Can you work these out from the model? Positions are in its coordinate system, mm. Round coordinates to 2 decimals unless told otherwise and drop trailing zeros. Return JSON: item names as keys, results as strings.
```python
from build123d import *

# Parameters (mm, degrees)
SKETCH_1_R      = 3.4
SKETCH_1_R_2    = 2
EXTRUDE_1_DEPTH = 1000


with BuildPart() as part:
    # 草图1 → 凸台-拉伸1 (new body)
    with BuildSketch(Plane.XY):
        with BuildLine():
            Line((5.39426949, 3.798904284), (9.399904408, 7.804539202))
            Line((9.399904408, 7.804539202), (12.09426949, 7.804539202))
            ThreePointArc((12.09426949, 7.804539202), (12.306401524, 7.716671237), (12.39426949, 7.504539202))
            Line((12.39426949, 7.504539202), (12.39426949, 3.954539202))
            ThreePointArc((12.39426949, 3.954539202), (12.482137455, 3.742407168), (12.69426949, 3.654539202))
            Line((12.69426949, 3.654539202), (13.59426949, 3.654539202))
            Line((13.59426949, 3.654539202), (13.59426949, 4.454539202))
            ThreePointArc((13.59426949, 4.454539202), (13.652848133, 4.595960558), (13.79426949, 4.654539202))
            Line((13.79426949, 4.654539202), (14.59426949, 4.654539202))
            Line((14.59426949, 4.654539202), (14.59426949, 12.054539202))
            ThreePointArc((14.59426949, 12.054539202), (13.862036443, 13.822306155), (12.09426949, 14.554539202))
            Line((12.09426949, 14.554539202), (4.69426949, 14.554539202))
            Line((4.69426949, 14.554539202), (4.69426949, 13.754539202))
            ThreePointArc((4.69426949, 13.754539202), (4.635690846, 13.613117846), (4.49426949, 13.554539202))
            Line((4.49426949, 13.554539202), (3.69426949, 13.554539202))
            Line((3.69426949, 13.554539202), (3.69426949, 12.654539202))
            ThreePointArc((3.69426949, 12.654539202), (3.782137455, 12.442407168), (3.99426949, 12.354539202))
            Line((3.99426949, 12.354539202), (7.54426949, 12.354539202))
            ThreePointArc((7.54426949, 12.354539202), (7.756401524, 12.266671237), (7.84426949, 12.054539202))
            Line((7.84426949, 12.054539202), (7.84426949, 9.360174121))
            Line((7.84426949, 9.360174121), (3.838634571, 5.354539202))
            Line((3.838634571, 5.354539202), (-4.650095592, 5.354539202))
            Line((-4.650095592, 5.354539202), (-8.65573051, 9.360174121))
            Line((-8.65573051, 9.360174121), (-8.65573051, 12.054539202))
            ThreePointArc((-8.65573051, 12.054539202), (-8.567862545, 12.266671237), (-8.35573051, 12.354539202))
            Line((-8.35573051, 12.354539202), (-4.80573051, 12.354539202))
            ThreePointArc((-4.80573051, 12.354539202), (-4.593598476, 12.442407168), (-4.50573051, 12.654539202))
            Line((-4.50573051, 12.654539202), (-4.50573051, 13.554539202))
            Line((-4.50573051, 13.554539202), (-5.30573051, 13.554539202))
            ThreePointArc((-5.30573051, 13.554539202), (-5.447151867, 13.613117846), (-5.50573051, 13.754539202))
            Line((-5.50573051, 13.754539202), (-5.50573051, 14.554539202))
            Line((-5.50573051, 14.554539202), (-12.90573051, 14.554539202))
            ThreePointArc((-12.90573051, 14.554539202), (-14.673497463, 13.822306155), (-15.40573051, 12.054539202))
            Line((-15.40573051, 12.054539202), (-15.40573051, 4.654539202))
            Line((-15.40573051, 4.654539202), (-14.60573051, 4.654539202))
            ThreePointArc((-14.60573051, 4.654539202), (-14.464309154, 4.595960558), (-14.40573051, 4.454539202))
            Line((-14.40573051, 4.454539202), (-14.40573051, 3.654539202))
            Line((-14.40573051, 3.654539202), (-13.50573051, 3.654539202))
            ThreePointArc((-13.50573051, 3.654539202), (-13.293598476, 3.742407168), (-13.20573051, 3.954539202))
            Line((-13.20573051, 3.954539202), (-13.20573051, 7.504539202))
            ThreePointArc((-13.20573051, 7.504539202), (-13.117862545, 7.716671237), (-12.90573051, 7.804539202))
            Line((-12.90573051, 7.804539202), (-10.211365429, 7.804539202))
            Line((-10.211365429, 7.804539202), (-6.20573051, 3.798904284))
            Line((-6.20573051, 3.798904284), (-6.20573051, -4.689825879))
            Line((-6.20573051, -4.689825879), (-10.211365429, -8.695460798))
            Line((-10.211365429, -8.695460798), (-12.90573051, -8.695460798))
            ThreePointArc((-12.90573051, -8.695460798), (-13.117862545, -8.607592832), (-13.20573051, -8.395460798))
            Line((-13.20573051, -8.395460798), (-13.20573051, -4.845460798))
            ThreePointArc((-13.20573051, -4.845460798), (-13.293598476, -4.633328763), (-13.50573051, -4.545460798))
            Line((-13.50573051, -4.545460798), (-14.40573051, -4.545460798))
            Line((-14.40573051, -4.545460798), (-14.40573051, -5.345460798))
            ThreePointArc((-14.40573051, -5.345460798), (-14.464309154, -5.486882154), (-14.60573051, -5.545460798))
            Line((-14.60573051, -5.545460798), (-15.40573051, -5.545460798))
            Line((-15.40573051, -5.545460798), (-15.40573051, -12.945460798))
            ThreePointArc((-15.40573051, -12.945460798), (-14.673497463, -14.713227751), (-12.90573051, -15.445460798))
            Line((-12.90573051, -15.445460798), (-5.50573051, -15.445460798))
            Line((-5.50573051, -15.445460798), (-5.50573051, -14.645460798))
            ThreePointArc((-5.50573051, -14.645460798), (-5.447151867, -14.504039442), (-5.30573051, -14.445460798))
            Line((-5.30573051, -14.445460798), (-4.50573051, -14.445460798))
            Line((-4.50573051, -14.445460798), (-4.50573051, -13.545460798))
            ThreePointArc((-4.50573051, -13.545460798), (-4.593598476, -13.333328763), (-4.80573051, -13.245460798))
            Line((-4.80573051, -13.245460798), (-8.35573051, -13.245460798))
            ThreePointArc((-8.35573051, -13.245460798), (-8.567862545, -13.157592832), (-8.65573051, -12.945460798))
            Line((-8.65573051, -12.945460798), (-8.65573051, -10.251095716))
            Line((-8.65573051, -10.251095716), (-4.650095592, -6.245460798))
            Line((-4.650095592, -6.245460798), (3.838634571, -6.245460798))
            Line((3.838634571, -6.245460798), (7.84426949, -10.251095716))
            Line((7.84426949, -10.251095716), (7.84426949, -12.945460798))
            ThreePointArc((7.84426949, -12.945460798), (7.756401524, -13.157592832), (7.54426949, -13.245460798))
            Line((7.54426949, -13.245460798), (3.99426949, -13.245460798))
            ThreePointArc((3.99426949, -13.245460798), (3.782137455, -13.333328763), (3.69426949, -13.545460798))
            Line((3.69426949, -13.545460798), (3.69426949, -14.445460798))
            Line((3.69426949, -14.445460798), (4.49426949, -14.445460798))
            ThreePointArc((4.49426949, -14.445460798), (4.635690846, -14.504039442), (4.69426949, -14.645460798))
            Line((4.69426949, -14.645460798), (4.69426949, -15.445460798))
            Line((4.69426949, -15.445460798), (12.09426949, -15.445460798))
            ThreePointArc((12.09426949, -15.445460798), (13.862036443, -14.713227751), (14.59426949, -12.945460798))
            Line((14.59426949, -12.945460798), (14.59426949, -5.545460798))
            Line((14.59426949, -5.545460798), (13.79426949, -5.545460798))
            ThreePointArc((13.79426949, -5.545460798), (13.652848133, -5.486882154), (13.59426949, -5.345460798))
            Line((13.59426949, -5.345460798), (13.59426949, -4.545460798))
            Line((13.59426949, -4.545460798), (12.69426949, -4.545460798))
            ThreePointArc((12.69426949, -4.545460798), (12.482137455, -4.633328763), (12.39426949, -4.845460798))
            Line((12.39426949, -4.845460798), (12.39426949, -8.395460798))
            ThreePointArc((12.39426949, -8.395460798), (12.306401524, -8.607592832), (12.09426949, -8.695460798))
            Line((12.09426949, -8.695460798), (9.399904408, -8.695460798))
            Line((9.399904408, -8.695460798), (5.39426949, -4.689825879))
            Line((5.39426949, -4.689825879), (5.39426949, 3.798904284))
        make_face()
        with Locations((-0.40573051, -0.445460798)):
            Circle(SKETCH_1_R, mode=Mode.SUBTRACT)
        with Locations((-12.03073051, 11.179539202)):
            Circle(SKETCH_1_R_2, mode=Mode.SUBTRACT)
        with Locations((11.21926949, 11.179539202)):
            Circle(SKETCH_1_R_2, mode=Mode.SUBTRACT)
        with Locations((-12.03073051, -12.070460798)):
            Circle(SKETCH_1_R_2, mode=Mode.SUBTRACT)
        with Locations((11.21926949, -12.070460798)):
            Circle(SKETCH_1_R_2, mode=Mode.SUBTRACT)
    extrude(amount=EXTRUDE_1_DEPTH)


solid = part.part
```
Q1. I'm going to push flat-ended pins straight in: pin 1 Ø0.6 at (y, z) = (-5, 558) entering from +X; pin 2 Ø0.7 at (x, z) = (13, 326) entering from +Y; pin 3 Ø0.6 at (y, z) = (-15, 647) entering from +X. Where does each tip first touch, or does it pass through?
Results:
{"pin 1": "stops at x = 13.59", "pin 2": "stops at y = 14.49", "pin 3": "stops at x = 13.88"}
Q2. If I drill on line 1 along Y through (x, z) = (-7, 174); line 2 along X through (y, z) = (-7, 76); line 3 along X through (y, z) = (-1.25, 235.5), over which ranges is the centre line in solid material (lowest first)?
Results:
{"line 1": "y = -15.45 to -13.25, -8.6 to -5.48, 4.59 to 7.7, 12.35 to 14.55", "line 2": "x = -15.41 to -13.21, -8.52 to -5.4, 4.59 to 7.7, 12.39 to 14.59", "line 3": "x = -6.21 to -3.71, 2.9 to 5.39"}
Q3. Suppose I cut it at A-A, the plane z = 120.5. State how many separate pieces and enclosed holes the cut face has, plus the area to 3 significant figures.
Results:
{"separate pieces": "1", "enclosed holes": "5", "area": "330 mm2"}
